Here's how the part is built. I have some questions about the finished solid (model axes, mm). A direction names the side the tool comes from. Round coordinates to 2 decimals unless told otherwise and drop trailing zeros. Write each loop counter-clockwise with the first axis right and the second up, starting at its lowest first coordinate (ties: lowest second). Pieces come first, ordered by that corner, then holes. Notation, with made-up numbers: (-19.5, -35) -> (-12.5, -35) arc R27 ccw to (-12.5, 4) -> close; hole circle Ø11 at (65.25, -25). An arc over 180 degrees is marked (long way). Answer as CSV lines item,"result".
```python
from build123d import *

# Parameters (mm, degrees)
SKETCH_1_R               = 30
SKETCH_1_R_2             = 2.75
EXTRUDE_1_DEPTH          = 5
SKETCH_2_R               = 12
EXTRUDE_2_DEPTH          = 10
SKETCH_3_R               = 6
EXTRUDE_3_DEPTH          = 10
SKETCH_4_R               = 5
EXTRUDE_4_DEPTH          = 8
SKETCH_5_R               = 4.9
EXTRUDE_5_DEPTH          = 1.1
SKETCH_6_R               = 5
EXTRUDE_6_DEPTH          = 15
CUT_EXTRUDE_1_DEPTH      = 15
CUT_EXTRUDE_1_DEPTH_BACK = 15
SKETCH_7_R               = 2


with BuildPart() as part:
    # Sketch 1 → Extrude 1 (new body)
    with BuildSketch(Plane.XY):
        Circle(SKETCH_1_R)
        with Locations((0, 22.5)):
            Circle(SKETCH_1_R_2, mode=Mode.SUBTRACT)
        with Locations((19.485571585, 11.25)):
            Circle(SKETCH_1_R_2, mode=Mode.SUBTRACT)
        with Locations((19.485571585, -11.25)):
            Circle(SKETCH_1_R_2, mode=Mode.SUBTRACT)
        with Locations((0, -22.5)):
            Circle(SKETCH_1_R_2, mode=Mode.SUBTRACT)
        with Locations((-19.485571585, -11.25)):
            Circle(SKETCH_1_R_2, mode=Mode.SUBTRACT)
        with Locations((-19.485571585, 11.25)):
            Circle(SKETCH_1_R_2, mode=Mode.SUBTRACT)
    extrude(amount=EXTRUDE_1_DEPTH)

    # Sketch 2 → Extrude 2 (add)
    with BuildSketch(Plane(origin=(0, 0, 0), x_dir=(-1, 0, 0), z_dir=(0, 0, -1))):
        with Locations(Location((0, 0, 0), (0, 0, 180))):
            Circle(SKETCH_2_R)
    extrude(amount=EXTRUDE_2_DEPTH)

    # Sketch 3 → Extrude 3 (add)
    with BuildSketch(Plane(origin=(0, 0, -10), x_dir=(-1, 0, 0), z_dir=(0, 0, -1))):
        Circle(SKETCH_3_R)
    extrude(amount=EXTRUDE_3_DEPTH)

    # Sketch 4 → Extrude 4 (add)
    with BuildSketch(Plane(origin=(0, 0, -20), x_dir=(-1, 0, 0), z_dir=(0, 0, -1))):
        Circle(SKETCH_4_R)
    extrude(amount=EXTRUDE_4_DEPTH)

    # Sketch 5 → Extrude 5 (add)
    with BuildSketch(Plane(origin=(0, 0, -28), x_dir=(-1, 0, 0), z_dir=(0, 0, -1))):
        Circle(SKETCH_5_R)
    extrude(amount=EXTRUDE_5_DEPTH)

    # Sketch 6 → Extrude 6 (add)
    with BuildSketch(Plane(origin=(0, 0, -29.1), x_dir=(-1, 0, 0), z_dir=(0, 0, -1))):
        Circle(SKETCH_6_R)
    extrude(amount=EXTRUDE_6_DEPTH)

    # Sketch 7 → Cut-Extrude 1 (cut, two sides: drawn at the far end of the back side and taken through both)
    with BuildSketch(Plane(origin=(0, 0, 0), x_dir=(1, 0, 0), z_dir=(0, 1, 0)).offset(-CUT_EXTRUDE_1_DEPTH_BACK)):
        with Locations(Location((0, 40.1, 0), (0, 0, 90))):
            Circle(SKETCH_7_R)
    extrude(amount=CUT_EXTRUDE_1_DEPTH + CUT_EXTRUDE_1_DEPTH_BACK, mode=Mode.SUBTRACT)


solid = part.part
```
1. For pin 1 Ø9 at (x, y) = (0, -22.5) entering from +Z; pin 2 Ø7 at (x, y) = (19.49, -11.25) entering from -Z; pin 3 Ø1 at (x, z) = (-2.5, 0) entering from -Y, each with a flat end and sliding along its axis, tell me the tip position at first contact or that it passes through.
Numbers:
pin 1,"stops at z = 5"
pin 2,"stops at z = 0"
pin 3,"stops at y = -29.93"
2. If we mould it in two halves opening along Z, with no side actions, what happens to faces 3 (the face through (-0.358, 25.227, 2.465)), 4 (the face through (1.062, -4.783, -28.542)), 5 (the face through (4, 4, -20))? For each: released by +Z, released by -Z, zero draft, split by the parting line, or undercut.
Numbers:
face 3,"zero draft"
face 4,"undercut"
face 5,"released by -Z"
3. Suppose I cut it at D-D on z = -5.5. Please give me the cut outline in (x, y), and give its area (3 significant figures).
Numbers:
outline,"circle Ø24 at (0, 0)"
area,"452 mm^2"
4. Suppose I cut it at B-B on x = -10. Please give me the cut outline in (y, z).
Numbers:
outline,"(-28.28, 0) -> (-6.63, 0) -> (-6.63, -10) -> (6.63, -10) -> (6.63, 0) -> (28.28, 0) -> (28.28, 5) -> (-28.28, 5) -> close"
5. Suppose I cut it at A-A on y = 22.5. Please give me the cut outline in (x, z), and give its area (3 significant figures).
Numbers:
outline,"(-19.84, 0) -> (-2.75, 0) -> (-2.75, 5) -> (-19.84, 5) -> close; (2.75, 0) -> (19.84, 0) -> (19.84, 5) -> (2.75, 5) -> close"
area,"171 mm^2"
6. On a 3-axis mill with a long thin cutter (end or side, diameter ignored), from which of +Z, -Z, +X, -X, +Y, -Y can I reach the whole of each face in a straight line? I mean faces 1 (the face through (0.766, -0.07, -41.947)), 2 (the face through (11.446, -3.604, -4.93)). Say none if no direction works.
Numbers:
face 1,"+Y, -Y"
face 2,"-Z"
7. Suppose I cut it at C-C on y = -4. Please give me the cut outline in (x, z).
Numbers:
outline,"(-29.73, 0) -> (-11.31, 0) -> (-11.31, -10) -> (-4.47, -10) -> (-4.47, -20) -> (-3, -20) -> (-3, -28) -> (-2.83, -28) -> (-2.83, -29.1) -> (-3, -29.1) -> (-3, -44.1) -> (3, -44.1) -> (3, -29.1) -> (2.83, -29.1) -> (2.83, -28) -> (3, -28) -> (3, -20) -> (4.47, -20) -> (4.47, -10) -> (11.31, -10) -> (11.31, 0) -> (29.73, 0) -> (29.73, 5) -> (-29.73, 5) -> close; hole circle Ø4 at (0, -40.1)"
8. If I drill on line 1 (Y direction, x = 0, z = 3.8); line 2 (Y direction, x = -22, z = 2.5); line 3 (X direction, y = 11, z = 2), over which ranges is the centre line in solid material (lowest first)?
Numbers:
line 1,"y = -30 to -25.25, -19.75 to 19.75, 25.25 to 30"
line 2,"y = -20.4 to -12.36, -10.14 to 10.14, 12.36 to 20.4"
line 3,"x = -27.91 to -22.22, -16.75 to 16.75, 22.22 to 27.91"
